from build123d import *

# Parameters (mm, degrees)
CHAMFER1_SIZE = 0.1
CHAMFER3_SIZE = 0.1
CHAMFER4_SIZE = 0.1
CHAMFER5_SIZE = 0.1


with BuildPart() as part:
    # Sketch1 → Revolve1 (revolve)
    with BuildSketch(Plane.XY, mode=Mode.PRIVATE) as revolve1_sk:
        Polygon((0, 0), (29, 0), (62, 0), (62, 2), (29, 2), (29, 3), (19, 3), (19, 2.125), (0, 2.125), align=None)
    revolve(revolve1_sk.sketch.rotate(Axis((0, 0, 0), (1, 0, 0)), 90), axis=Axis((0, 0, 0), (1, 0, 0)))

    # Chamfer1
    chamfer1_edges = [part.edges().sort_by_distance(p)[0] for p in [
        (0, 0, -2.125),
    ]]
    chamfer(chamfer1_edges, length=CHAMFER1_SIZE)

    # Chamfer3
    chamfer3_edges = [part.edges().sort_by_distance(p)[0] for p in [
        (29, 0, -3),
    ]]
    chamfer(chamfer3_edges, length=CHAMFER3_SIZE)

    # Chamfer4
    chamfer4_edges = [part.edges().sort_by_distance(p)[0] for p in [
        (62, 0, -2),
    ]]
    chamfer(chamfer4_edges, length=CHAMFER4_SIZE)

    # Chamfer5
    chamfer5_edges = [part.edges().sort_by_distance(p)[0] for p in [
        (19, 0, -3),
    ]]
    chamfer(chamfer5_edges, length=CHAMFER5_SIZE)


solid = part.part
Geometry check sheet. Reference: the model listing, model coordinates, mm. A direction names the side the tool comes from. Coordinates: 2 decimals unless noted, no trailing zeros. Order: outer loops, then holes, each group sorted by start corner. A loop starts at its lowest first (then second) coordinate and runs counter-clockwise, first axis right, second up. Notation, with made-up numbers: (34.5, 7) -> (61.5, 7) arc R14 ccw to (61.5, 31) -> close; hole circle Ø5 at (7, 41). An arc over 180 degrees is marked (long way). Use a Markdown table: item, result. Add a question column.
1. Go/stop test with flat-tipped pins: pin 1 Ø2 at (x, z) = (47, -0.5) entering from +Y; pin 2 Ø1.5 at (x, y) = (46, -2) entering from +Z; pin 3 Ø3 at (x, z) = (11.5, -1) entering from -Y (3 decimals). Record where each tip stops, or that it passes through.
2. Cross-section at A-A (z = 0). Enter the section's corners in (x, y) (3 decimals).
3. Material ranges on L1, parallel to Z at x = 9.5, y = -0.2; L2, parallel to X at y = 2.3, z = 1.3; L3, parallel to Y at x = 56.5, z = -0.2, recorded low to high.
4. Cross-section at C-C (x = 12.5). Enter the section's corners in (y, z) (3 decimals).
5. Set-up check for faces 4 (the face through (62, 0, 0)), 5 (the face through (45, 2, 0)): record each of +Z, -Z, +X, -X, +Y, -Y from which the full face is reachable in a straight line by a thin tool's end or side.
6. Cross-section at D-D (x = 27). Enter the section's corners in (y, z), and give its area (3 significant figures).
7. Mould release check, pull along X, two halves, no side actions. Record for faces 1 (the face through (9.418, -2.107, -0.277)), 2 (the face through (0, 0, 0)), 3 (the face through (29, 2, 1)): pulls with the +X half, pulls with the -X half, needs draft (parallel to the pull), parting line crosses it, or undercut.
Filled sheet:
| question | item | result |
|---|---|---|
| 1 | pin 1 | y = 2 |
| 1 | pin 2 | z = 1.56 |
| 1 | pin 3 | y = -2.125 |
| 2 | outline | (0, -2.025) -> (0.1, -2.125) -> (19, -2.125) -> (19, -2.9) -> (19.1, -3) -> (28.9, -3) -> (29, -2.9) -> (29, -2) -> (61.9, -2) -> (62, -1.9) -> (62, 1.9) -> (61.9, 2) -> (29, 2) -> (29, 2.9) -> (28.9, 3) -> (19.1, 3) -> (19, 2.9) -> (19, 2.125) -> (0.1, 2.125) -> (0, 2.025) -> close |
| 3 | L1 | -2.12 to 2.12 |
| 3 | L2 | 19 to 29 |
| 3 | L3 | -1.99 to 1.99 |
| 4 | outline | circle Ø4.25 at (0, 0) |
| 5 | face 4 | +Z, -Z, +X, +Y, -Y |
| 5 | face 5 | +X |
| 6 | outline | circle Ø6 at (0, 0) |
| 6 | area | 28.3 mm2 |
| 7 | face 1 | needs draft |
| 7 | face 2 | pulls with the -X half |
| 7 | face 3 | pulls with the +X half |
